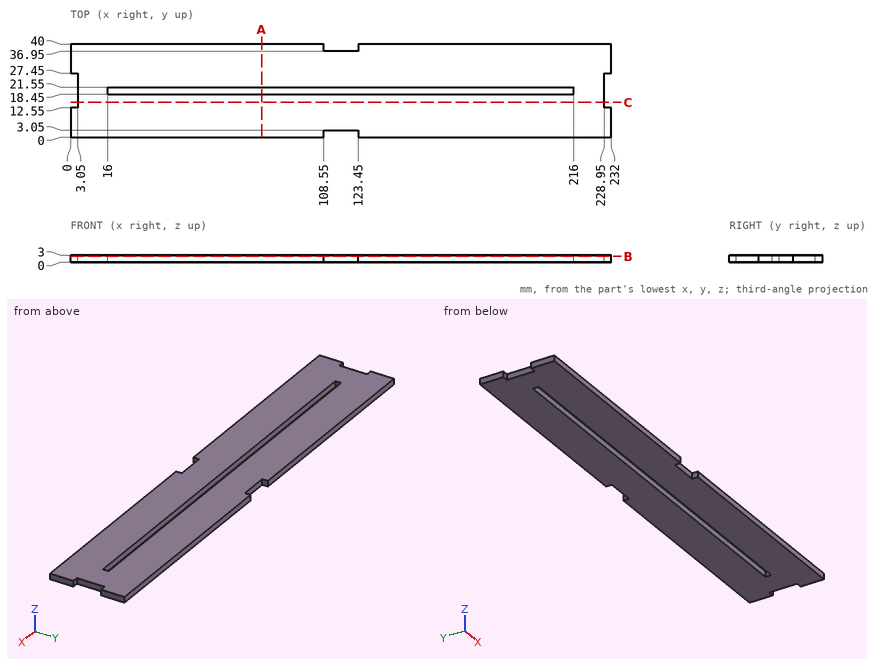
For this review, use the dimensioned drawing (mm, ordinates from the lowest corner) and the shaded views. Give positions to 0.01 mm unless a question says otherwise; leave off trailing zeros. Loops run counter-clockwise (first coordinate to the right, second up) from the corner with the lowest first, then second, coordinate; pieces in that order, holes last.
Item 1: Take a section at C-C, the plane y = 15. State the section outline as (x, z) points, and give its area (3 significant figures).
Item 2: Take a section at A-A, the plane x = 82. State the section outline as (y, z) points.
Item 3: For line 1 along X through (y, z) = (19.5, 2.65); line 2 along Y through (x, z) = (50, 2.2); line 3 along Y through (x, z) = (113, 0.25), list the stretches that pass through material, from the lowest coordinate up.
Item 4: Take a section at B-B, the plane z = 2.55. State the section outline as (x, y) points.
Item 5: Insertion check: pin 1 (1.5 mm diameter, centred on x = 119.5, z = 1.5, fed in from -Y); pin 2 (1 mm diameter, centred on y = 7, z = 0.5, fed in from -X); pin 3 (0.9 mm diameter, centred on y = 16.5, z = 1, fed in from -X); pin 4 (1.5 mm diameter, centred on y = 19.5, z = 1.5, fed in from +X). Each pin has a flat end and moves straight along its axis. Give the tip position at first contact, or say it passes through.
Calculated:
1. outline: (3.05, 0) - (228.95, 0) - (228.95, 3) - (3.05, 3) - close
1. area: 678 mm2
2. outline: (0, 0) - (18.45, 0) - (18.45, 3) - (0, 3) - close; (21.55, 0) - (40, 0) - (40, 3) - (21.55, 3) - close
3. line 1: x = 3.05 to 16, 216 to 228.95
3. line 2: y = 0 to 18.45, 21.55 to 40
3. line 3: y = 3.05 to 18.45, 21.55 to 36.95
4. outline: (0, 0) - (108.55, 0) - (108.55, 3.05) - (123.45, 3.05) - (123.45, 0) - (232, 0) - (232, 12.55) - (228.95, 12.55) - (228.95, 27.45) - (232, 27.45) - (232, 40) - (123.45, 40) - (123.45, 36.95) - (108.55, 36.95) - (108.55, 40) - (0, 40) - (0, 27.45) - (3.05, 27.45) - (3.05, 12.55) - (0, 12.55) - close; hole (16, 18.45) - (216, 18.45) - (216, 21.55) - (16, 21.55) - close
5. pin 1: stops at y = 3.05
5. pin 2: stops at x = 0
5. pin 3: stops at x = 3.05
5. pin 4: stops at x = 228.95
